```python
from build123d import *

# Parameters (mm, degrees)
SKETCH1_W                       = 116
SKETCH1_H                       = 42
BOSS_EXTRUDE1_DEPTH             = 7
BOSS_EXTRUDE2_REACH             = 64.081
SKETCH2_R                       = 1.75
BOSS_EXTRUDE2_DIRECTION_2_REACH = 64.081
SKETCH2_3_R                     = 1.75
CUT_EXTRUDE1_DEPTH              = 54
BOSS_EXTRUDE3_DEPTH             = 25
FILLET1_R                       = 3


with BuildPart() as part:
    # Sketch1 → Boss-Extrude1 (new body)
    with BuildSketch(Plane(origin=(0, 0, 0), x_dir=(1, 0, 0), z_dir=(0, 1, 0))):
        Rectangle(SKETCH1_W, SKETCH1_H)
    extrude(amount=BOSS_EXTRUDE1_DEPTH)

    # Boss-Extrude2: up to this face of the body (flat: up to its plane)
    boss_extrude2_end = Plane(part.part.faces().sort_by_distance((58, 3.5, 0))[0])
    # Sketch2 → Boss-Extrude2 (add, up to the picked face)
    with BuildSketch(Plane(origin=(0, 0, 0), x_dir=(0, 0, -1), z_dir=(1, 0, 0)), mode=Mode.PRIVATE) as boss_extrude2_sk1:
        with BuildLine():
            ThreePointArc((10, 13), (8.586149806, 9.094875162), (5, 7))
            Line((5, 7), (10, 7))
            Line((10, 7), (21, 7))
            Line((21, 7), (21, 18))
            Line((21, 18), (15, 18))
            ThreePointArc((15, 18), (11.464466094, 16.535533906), (10, 13))
        make_face()
        with Locations(Location((15.5, 12.475, 0), (0, 0, 180))):
            Circle(SKETCH2_R, mode=Mode.SUBTRACT)
    boss_extrude2_tool1 = split(extrude(boss_extrude2_sk1.sketch, amount=BOSS_EXTRUDE2_REACH, mode=Mode.PRIVATE), bisect_by=boss_extrude2_end, keep=Keep.BOTH, mode=Mode.PRIVATE)
    # Sketch2 → Boss-Extrude2 (add, up to the picked face)
    with BuildSketch(Plane(origin=(0, 0, 0), x_dir=(0, 0, -1), z_dir=(1, 0, 0)), mode=Mode.PRIVATE) as boss_extrude2_sk2:
        with BuildLine():
            Line((-21, 18), (-21, 7))
            Line((-21, 7), (-5, 7))
            ThreePointArc((-5, 7), (-8.586149806, 9.094875162), (-10, 13))
            ThreePointArc((-10, 13), (-11.464466094, 16.535533906), (-15, 18))
            Line((-15, 18), (-21, 18))
        make_face()
        with Locations(Location((-15.5, 12.475, 0), (0, 0, 180))):
            Circle(SKETCH2_R, mode=Mode.SUBTRACT)
    boss_extrude2_tool2 = split(extrude(boss_extrude2_sk2.sketch, amount=BOSS_EXTRUDE2_REACH, mode=Mode.PRIVATE), bisect_by=boss_extrude2_end, keep=Keep.BOTH, mode=Mode.PRIVATE)
    add(boss_extrude2_tool1.solids().sort_by(Axis((0, 8.970574, -8.735311), (1, 0, 0)))[0])
    add(boss_extrude2_tool2.solids().sort_by(Axis((0, 12.5, 20.805835), (1, 0, 0)))[0])

    # Boss-Extrude2 direction 2: up to this face of the body (flat: up to its plane)
    boss_extrude2_direction_2_end = Plane(part.part.faces().sort_by_distance((-58, 3.5, 0))[0])
    # Sketch2 → Boss-Extrude2 direction 2 (add, up to the picked face)
    with BuildSketch(Plane(origin=(0, 0, 0), x_dir=(0, 0, -1), z_dir=(1, 0, 0)), mode=Mode.PRIVATE) as boss_extrude2_direction_2_sk1:
        with BuildLine():
            ThreePointArc((10, 13), (8.586149806, 9.094875162), (5, 7))
            Line((5, 7), (10, 7))
            Line((10, 7), (21, 7))
            Line((21, 7), (21, 18))
            Line((21, 18), (15, 18))
            ThreePointArc((15, 18), (11.464466094, 16.535533906), (10, 13))
        make_face()
        with Locations(Location((15.5, 12.475, 0), (0, 0, 180))):
            Circle(SKETCH2_R, mode=Mode.SUBTRACT)
    boss_extrude2_direction_2_tool1 = split(extrude(boss_extrude2_direction_2_sk1.sketch, amount=-BOSS_EXTRUDE2_DIRECTION_2_REACH, mode=Mode.PRIVATE), bisect_by=boss_extrude2_direction_2_end, keep=Keep.BOTH, mode=Mode.PRIVATE)
    # Sketch2 → Boss-Extrude2 direction 2 (add, up to the picked face)
    with BuildSketch(Plane(origin=(0, 0, 0), x_dir=(0, 0, -1), z_dir=(1, 0, 0)), mode=Mode.PRIVATE) as boss_extrude2_direction_2_sk2:
        with BuildLine():
            Line((-21, 18), (-21, 7))
            Line((-21, 7), (-5, 7))
            ThreePointArc((-5, 7), (-8.586149806, 9.094875162), (-10, 13))
            ThreePointArc((-10, 13), (-11.464466094, 16.535533906), (-15, 18))
            Line((-15, 18), (-21, 18))
        make_face()
        with Locations(Location((-15.5, 12.475, 0), (0, 0, 180))):
            Circle(SKETCH2_R, mode=Mode.SUBTRACT)
    boss_extrude2_direction_2_tool2 = split(extrude(boss_extrude2_direction_2_sk2.sketch, amount=-BOSS_EXTRUDE2_DIRECTION_2_REACH, mode=Mode.PRIVATE), bisect_by=boss_extrude2_direction_2_end, keep=Keep.BOTH, mode=Mode.PRIVATE)
    add(boss_extrude2_direction_2_tool1.solids().sort_by(Axis((0, 8.970574, -8.735311), (-1, 0, 0)))[0])
    add(boss_extrude2_direction_2_tool2.solids().sort_by(Axis((0, 12.5, 20.805835), (-1, 0, 0)))[0])

    # Sketch2_3 → Cut-Extrude1 (cut, symmetric)
    # profile 1 of 2: a face of its own
    with BuildSketch(Plane(origin=(0, 0, 0), x_dir=(0, 0, -1), z_dir=(1, 0, 0))):
        with BuildLine():
            ThreePointArc((10, 13), (8.586149806, 9.094875162), (5, 7))
            Line((5, 7), (10, 7))
            Line((10, 7), (21, 7))
            Line((21, 7), (21, 18))
            Line((21, 18), (15, 18))
            ThreePointArc((15, 18), (11.464466094, 16.535533906), (10, 13))
        make_face()
        with Locations((15.5, 12.475)):
            Circle(SKETCH2_3_R, mode=Mode.SUBTRACT)
    # profile 2 of 2: a face of its own
    with BuildSketch(Plane(origin=(0, 0, 0), x_dir=(0, 0, -1), z_dir=(1, 0, 0))):
        with BuildLine():
            Line((-21, 18), (-21, 7))
            Line((-21, 7), (-5, 7))
            ThreePointArc((-5, 7), (-8.586149806, 9.094875162), (-10, 13))
            ThreePointArc((-10, 13), (-11.464466094, 16.535533906), (-15, 18))
            Line((-15, 18), (-21, 18))
        make_face()
        with Locations((-15.5, 12.475)):
            Circle(SKETCH2_3_R, mode=Mode.SUBTRACT)
    extrude(amount=CUT_EXTRUDE1_DEPTH, both=True, mode=Mode.SUBTRACT)

    # Sketch3 → Boss-Extrude3 (add)
    with BuildSketch(Plane(origin=(-54, 0, 0), x_dir=(0, 0, -1), z_dir=(1, 0, 0))):
        with BuildLine():
            Line((-21, 7), (-15, 7))
            ThreePointArc((-15, 7), (-18.465513805, 9.534486195), (-21, 13))
            Line((-21, 13), (-21, 7))
        make_face()
        with BuildLine():
            Line((21, 7), (21, 13))
            ThreePointArc((21, 13), (18.465513805, 9.534486195), (15, 7))
            Line((15, 7), (21, 7))
        make_face()
    boss_extrude3 = extrude(amount=BOSS_EXTRUDE3_DEPTH)

    # Mirror4: Boss-Extrude3 across plane
    add(boss_extrude3.mirror(Plane(origin=(0, 0, 0), x_dir=(0, 0, 1), z_dir=(1, 0, 0))))

    # Fillet1
    fillet1_edges = [part.edges().sort_by_distance(p)[0] for p in [
        (0, 0, 21),
        (0, 0, -21),
    ]]
    fillet(fillet1_edges, radius=FILLET1_R)


solid = part.part
```
The listing builds one solid part. Answer for the finished solid, in the listing's coordinates (mm). A direction names the side the tool comes from. Give positions to 0.01 mm unless a question says otherwise; leave off trailing zeros. Order: outer loops, then holes, each group sorted by start corner. A loop starts at its lowest first (then second) coordinate and runs counter-clockwise, first axis right, second up.
Item 1: Given pin 1 Ø6 at (x, z) = (24.5, -6) entering from +Y, flat-ended and moving along its own axis, determine where the tip first touches the part or whether it passes through.
From the geometry:
pin 1: stops at y = 7
Item 2: Find the intervals of material crossed by probe 1 along Y at (x, z) = (-56.8, -15.5) (3 decimals); probe 2 along X at (y, z) = (14.5, 14); probe 3 along Y at (x, z) = (-11.5, 15), in increasing order.
From the geometry:
probe 1: y = 0 to 10.725, 14.225 to 18
probe 2: x = -58 to -54, 54 to 58
probe 3: y = 0 to 7
Item 3: The part is cut by section D-D, the plane z = -4. Give the vertices of the cut face in (x, y), and give its area (3 significant figures).
From the geometry:
outline: (-58, 0) - (58, 0) - (58, 7) - (-58, 7) - close
area: 812 mm2
Item 4: The part is cut by section C-C, the plane x = -21. Give the vertices of the cut face in (y, z).
From the geometry:
outline: (0, -18) arc R3 ccw to (3, -21) - (7, -21) - (7, 21) - (3, 21) arc R3 ccw to (0, 18) - close
Item 5: Which of the six approach directions +Z, -Z, +X, -X, +Y, -Y give full straight-line access (tool end or side, diameter ignored) to faces 3 (the face through (0.81, 0.9, 20.14)), 4 (the face through (-29, 9, 19)), 5 (the face through (-54, 13, 13)), 6 (the face through (56, 17, -12)), 7 (the face through (1, 6, 21))?
From the geometry:
face 3: +Z, +X, -X, -Y
face 4: +Z, -Z, +Y
face 5: +Y
face 6: +X, -X, +Y
face 7: +Z, +X, -X, +Y, -Y
Item 6: The part is cut by section A-A, the plane z = -9. Give the vertices of the cut face in (x, y).
From the geometry:
outline: (-58, 0) - (58, 0) - (58, 9.65) - (54, 9.65) - (54, 7) - (-54, 7) - (-54, 9.65) - (-58, 9.65) - close
Item 7: For a pull along X with two mould halves and no side action, classify faces 1 (the face through (56.028, 13.145, -13.883)), 2 (the face through (41.68, 9.49, 18.42)) as pulls with the +X half, pulls with the -X half, needs draft (parallel to the pull), parting line crosses it, or undercut.
From the geometry:
face 1: needs draft
face 2: undercut
Item 8: The part is cut by section B-B, the plane x = 37. Give the vertices of the cut face in (y, z), and give its area (3 significant figures).
From the geometry:
outline: (0, -18) arc R3 ccw to (3, -21) - (13, -21) arc R14 cw to (7, -15) - (7, 15) arc R14 cw to (13, 21) - (3, 21) arc R3 ccw to (0, 18) - close
area: 319 mm2
